```python
from build123d import *

# Parameters (mm, degrees)
F0_R     = 10.5156
F1_DEPTH = 2.159
F2_R     = 5.4991
F3_DEPTH = 2.4384
F4_R     = 4.0894
F5_DEPTH = 5.588
F6_T     = -1.3716


with BuildPart() as f1:
    # F0 (on Top) → F1 (new body)
    with BuildSketch(Plane.XY):
        Circle(F0_R)
    extrude(amount=F1_DEPTH)

    # F2 (on Top) → F3 (join)
    with BuildSketch(Plane.XY):
        Circle(F2_R)
    extrude(amount=F3_DEPTH)

    # F4 (on Top) → F5 (join)
    with BuildSketch(Plane.XY):
        Circle(F4_R)
    extrude(amount=F5_DEPTH)

    # F6
    f6_openings = [f1.faces().sort_by_distance(p)[0] for p in [
        (0, 0, 5.588),
    ]]
    offset(amount=F6_T, openings=f6_openings, kind=Kind.INTERSECTION)


solid = f1.part
```
Can you work these out from the model? Positions are in its coordinate system, mm. A direction names the side the tool comes from. Round coordinates to 2 decimals unless told otherwise and drop trailing zeros. Loops run counter-clockwise (first coordinate to the right, second up) from the corner with the lowest first, then second, coordinate; pieces in that order, holes last. Notation, with made-up numbers: M 8.5,-21 L 62.5,-21 A32 cw 62.5,8 Z; hole C -36.5,-5 d4. An arc over 180 degrees is marked long. Answer as a JSON object with one key per item and string values. Group by question number.
Q1. Please list where these lines run through material, in increasing order: L1, parallel to Y at x = 0, z = 3.05; L2, parallel to Z at x = -5, y = -5.25.
Q2. Imagine slicing it at A-A, the plane x = 0. Please give me the cut outline in (y, z).
Q3. Will these pins go through, and if not, where does the flat tip stop? pin 1 (1.5 mm diameter, centred on y = 8.5, z = 0.5, fed in from +X); pin 2 (3.5 mm diameter, centred on x = 0, y = 0, fed in from +Z).
Q4. On a 3-axis mill with a long thin cutter (end or side, diameter ignored), from which of +Z, -Z, +X, -X, +Y, -Y can I reach the whole of each face in a straight line? I mean faces 4 (the cylindrical face through (10.03, 3.16, 1.06)), 5 (the cylindrical face through (-2.16, -1.65, 3.45)). Say none if no direction works.
Q5. We'd pull the mould along Y, two halves only. Please class faces 1 (the flat face through (0, 0, 1.372)), 2 (the flat face through (-4, -2, 2.438)), 3 (the cylindrical face through (3.9, 1.23, 3.99)): +Y half, -Y half, draft (parallel to the pull), parting line (faces both ways), or undercut.
Q6. Imagine slicing it at B-B, the plane z = 5. Please give me the cut outline in (x, y), then the cut area to 3 significant figures.
Q7. Imagine slicing it at D-D, the plane x = -5. Please give me the cut outline in (y, z).
Findings:
{
 "1": {"L1": "y = -4.09 to -2.72, 2.72 to 4.09", "L2": "z = 0 to 2.16"},
 "2": {"outline": "M -10.52,0 L 10.52,0 L 10.52,2.16 L 5.5,2.16 L 5.5,2.44 L 4.09,2.44 L 4.09,5.59 L 2.72,5.59 L 2.72,1.37 L -2.72,1.37 L -2.72,5.59 L -4.09,5.59 L -4.09,2.44 L -5.5,2.44 L -5.5,2.16 L -10.52,2.16 Z"},
 "3": {"pin 1": "stops at x = 7.11", "pin 2": "stops at z = 1.37"},
 "4": {"face 4": "+Z, -Z", "face 5": "+Z"},
 "5": {"face 1": "undercut", "face 2": "draft", "face 3": "parting line"},
 "6": {"outline": "C 0,0 d8.18; hole C 0,0 d5.44", "area": "29.3 mm2"},
 "7": {"outline": "M -9.25,0 L 9.25,0 L 9.25,2.16 L 2.29,2.16 L 2.29,2.44 L -2.29,2.44 L -2.29,2.16 L -9.25,2.16 Z"}
}
